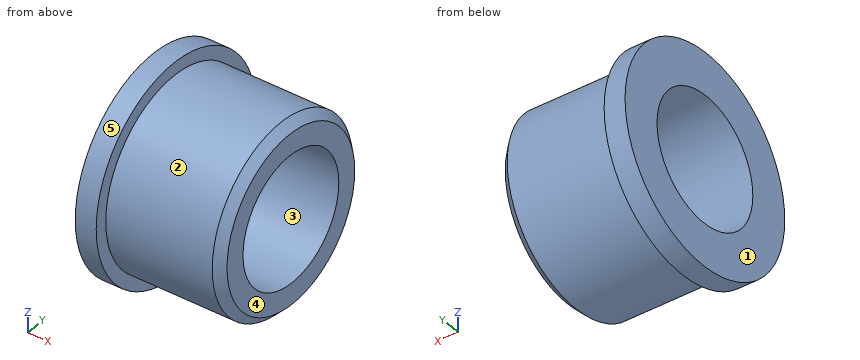
```python
from build123d import *

# Parameters (mm, degrees)
F2_SIZE = 1


with BuildPart() as f1:
    # F0 (on Top) → F1 (revolve)
    with BuildSketch(Plane.XY):
        Polygon((0, 12.5), (0, 7.5), (16.2, 7.5), (16.2, 11), (2.5, 11), (2.5, 12.5), align=None)
    revolve(axis=Axis((6.446342, 0, 0), (1, 0, 0)))

    # F2
    f2_edges = [f1.edges().sort_by_distance(p)[0] for p in [
        (16.2, -11, 0),
    ]]
    chamfer(f2_edges, length=F2_SIZE)


solid = f1.part
```
Geometry: final body of the model. Coordinates: model frame, mm. Face numbers are marked on the shaded views. A direction names the side the tool comes from. Coordinates: 2 decimals unless noted, no trailing zeros. Write each loop counter-clockwise with the first axis right and the second up, starting at its lowest first coordinate (ties: lowest second). Pieces come first, ordered by that corner, then holes. Notation, with made-up numbers: M 75,28 L 130,28 A29 cw 130,58 Z; hole C -4.5,-38.75 d10. An arc over 180 degrees is marked long. Answer as CSV lines item,"result". Start each with the question number.
Q1. Line query: line 1 (Z direction, x = 10, y = 0); line 2 (Y direction, x = 2, z = 5.75); line 3 (Y direction, x = 13.25, z = 5). Output: solid intervals per line, ascending. Write a range as from..to.
Q2. Cut plane A-A on z = 0. Return the cut outline in (x, y), then the cut area to 3 significant figures.
Q3. Cut plane C-C on x = 6. Return the cut outline in (y, z).
Q4. Reachability of the marked faces 1 and 2 from +Z, -Z, +X, -X, +Y, -Y: full face, straight path, thin tool, end or side. Return the list, or none.
Q5. Mould query, pull axis Z, two halves, no side actions, for the marked faces 3, 4 and 5. Classes: released by +Z, released by -Z, zero draft, split by the parting line, or undercut.
Q6. Pin query (flat end, axial travel): P1, Ø3, axis at x = 14, z = -9, coming from the -Y side; P2, Ø1.5, axis at x = 12, y = 0.5, coming from the +Z side; P3, Ø1, axis at x = 10, z = 2.5, coming from the -Y side; P4, Ø7.5, axis at y = 1, z = 1.5, coming from the +X side. Return the tip coordinate at first contact, or that it passes through.
Findings below:
1,line 1,"z = -11..-7.5, 7.5..11"
1,line 2,"y = -11.1..-4.82, 4.82..11.1"
1,line 3,"y = -9.8..-5.59, 5.59..9.8"
2,outline,"M 0,-12.5 L 2.5,-12.5 L 2.5,-11 L 15.2,-11 L 16.2,-10 L 16.2,-7.5 L 0,-7.5 Z; M 0,7.5 L 16.2,7.5 L 16.2,10 L 15.2,11 L 2.5,11 L 2.5,12.5 L 0,12.5 Z"
2,area,"120 mm2"
3,outline,"C 0,0 d22; hole C 0,0 d15"
4,face 1,"+Z, -Z, -X, +Y, -Y"
4,face 2,"+X"
5,face 3,"undercut"
5,face 4,"zero draft"
5,face 5,"split by the parting line"
6,P1,"stops at y = -8.05"
6,P2,"stops at z = 11"
6,P3,"stops at y = -10.82"
6,P4,"passes through"
